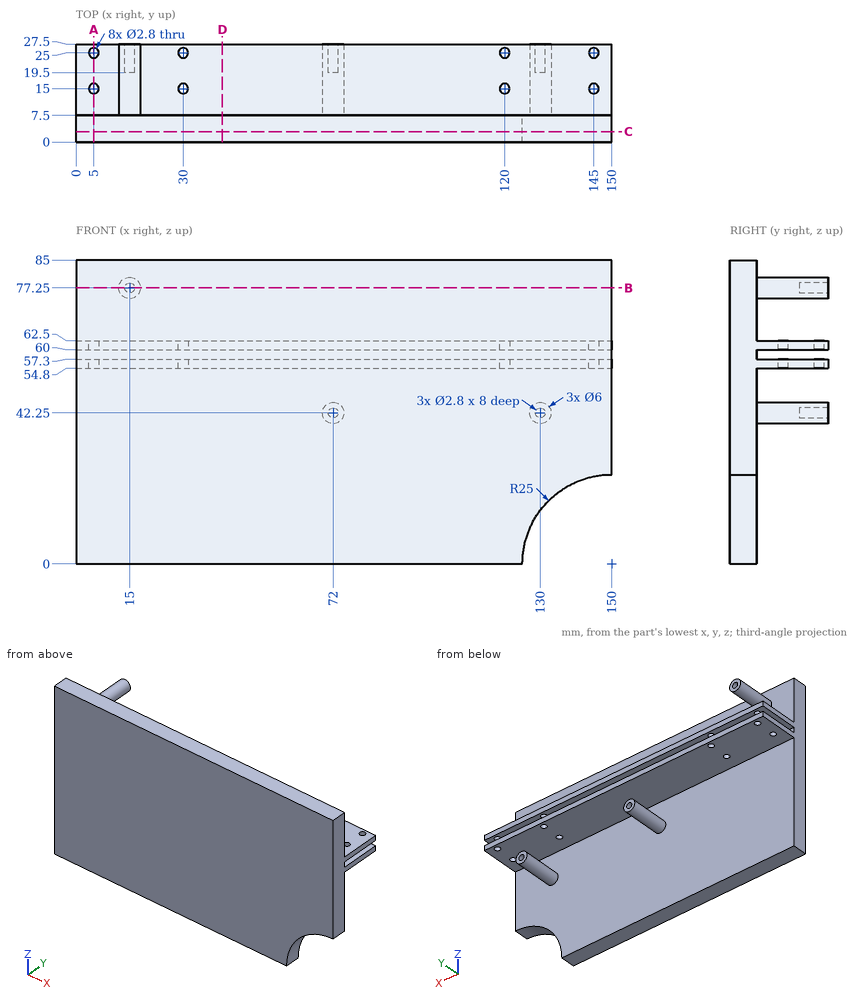
Print and shaded views of the part. All mm, measured from the part's lowest x, y and z. Give positions to 0.01 mm unless a question says otherwise; leave off trailing zeros. Loops run counter-clockwise (first coordinate to the right, second up) from the corner with the lowest first, then second, coordinate; pieces in that order, holes last. Notation, with made-up numbers: (23.25, 62) -> (50.25, 62) arc R31 cw to (50.25, 98) -> close; hole circle Ø10 at (5.25, 28). An arc over 180 degrees is marked (long way). One line per question, with ' | ' between items. Start each with the question number.
1) Pin check, flat tips, straight feed: pin 1 (3 mm diameter, centred on x = 5, y = 15, fed in from -Z); pin 2 (2.5 mm diameter, centred on x = 72, z = 42.25, fed in from +Y); pin 3 (4.5 mm diameter, centred on x = 120, y = 25, fed in from +Z); pin 4 (2 mm diameter, centred on x = 18, z = 12.5, fed in from -Y). Stop position of each tip, or through.
2) Cut at B-B (z = 77.25). Give the cut face in (x, y), plus the area to 3 significant figures.
3) Cut at C-C (y = 3). Give the cut face in (x, z).
4) Probe L1, parallel to Z at x = 63, y = 25; L2, parallel to Y at x = 5, z = 55.5; L3, parallel to Z at x = 130, y = 23.5. List the from-to ranges inside material, lowest first.
5) Cut at D-D (x = 41). Give the cut face in (y, z), plus the area to 4 significant figures.
6) Cut at A-A (x = 5). Give the cut face in (y, z), plus the area to 4 significant figures.
Return value:
1) pin 1: z = 54.8 | pin 2: y = 19.5 | pin 3: z = 62.5 | pin 4: y = 0
2) outline: (0, 0) -> (150, 0) -> (150, 7.5) -> (18, 7.5) -> (18, 27.5) -> (16.4, 27.5) -> (16.4, 19.5) -> (13.6, 19.5) -> (13.6, 27.5) -> (12, 27.5) -> (12, 7.5) -> (0, 7.5) -> close | area: 1,220 mm^2
3) outline: (0, 0) -> (125, 0) arc R25 cw to (150, 25) -> (150, 85) -> (0, 85) -> close
4) L1: 54.8 to 57.3, 60 to 62.5 | L2: 0 to 13.6, 16.4 to 23.6, 26.4 to 27.5 | L3: 39.25 to 40.85, 43.65 to 45.25, 54.8 to 57.3, 60 to 62.5
5) outline: (0, 0) -> (7.5, 0) -> (7.5, 54.8) -> (27.5, 54.8) -> (27.5, 57.3) -> (7.5, 57.3) -> (7.5, 60) -> (27.5, 60) -> (27.5, 62.5) -> (7.5, 62.5) -> (7.5, 85) -> (0, 85) -> close | area: 737.5 mm^2
6) outline: (0, 0) -> (7.5, 0) -> (7.5, 54.8) -> (13.6, 54.8) -> (13.6, 57.3) -> (7.5, 57.3) -> (7.5, 60) -> (13.6, 60) -> (13.6, 62.5) -> (7.5, 62.5) -> (7.5, 85) -> (0, 85) -> close; (16.4, 54.8) -> (23.6, 54.8) -> (23.6, 57.3) -> (16.4, 57.3) -> close; (16.4, 60) -> (23.6, 60) -> (23.6, 62.5) -> (16.4, 62.5) -> close; (26.4, 54.8) -> (27.5, 54.8) -> (27.5, 57.3) -> (26.4, 57.3) -> close; (26.4, 60) -> (27.5, 60) -> (27.5, 62.5) -> (26.4, 62.5) -> close | area: 709.5 mm^2
